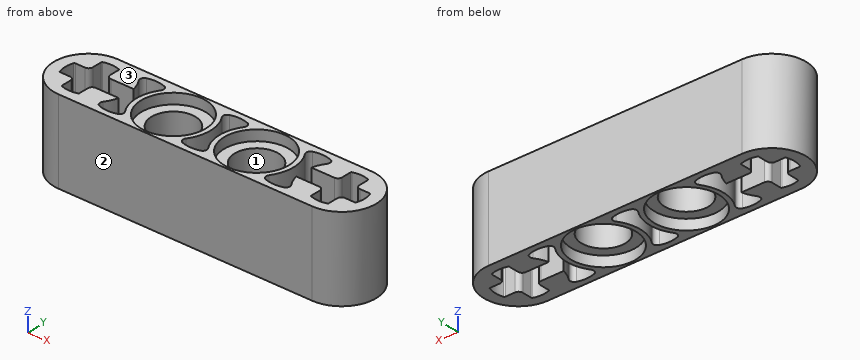
from build123d import *

# Parameters (mm, degrees)
SKETCH1_R           = 2.1
BOSS_EXTRUDE1_DEPTH = 4
SKETCH2_R           = 3.1
CUT_EXTRUDE1_DEPTH  = 1


with BuildPart() as part:
    # Sketch1 → Boss-Extrude1 (new, symmetric)
    with BuildSketch(Plane.XY):
        with BuildLine():
            Line((12.2, 3.3), (-12.2, 3.3))
            ThreePointArc((-12.2, 3.3), (-15.5, 0), (-12.2, -3.3))
            Line((-12.2, -3.3), (12.2, -3.3))
            ThreePointArc((12.2, -3.3), (15.5, 0), (12.2, 3.3))
        make_face()
        with BuildLine():
            Line((-14.177705214, 0.84), (-13.24, 0.84))
            ThreePointArc((-13.24, 0.84), (-12.957157288, 0.957157288), (-12.84, 1.24))
            Line((-12.84, 1.24), (-12.84, 2.177705214))
            ThreePointArc((-12.84, 2.177705214), (-12.821293884, 2.235940121), (-12.772173913, 2.27238805))
            ThreePointArc((-12.772173913, 2.27238805), (-12, 2.4), (-11.227826087, 2.27238805))
            ThreePointArc((-11.227826087, 2.27238805), (-11.178706116, 2.235940121), (-11.16, 2.177705214))
            Line((-11.16, 2.177705214), (-11.16, 1.24))
            ThreePointArc((-11.16, 1.24), (-11.042842712, 0.957157288), (-10.76, 0.84))
            Line((-10.76, 0.84), (-9.822294786, 0.84))
            Line((-9.822294786, 0.84), (-9.751800721, 0.84))
            Line((-9.751800721, 0.84), (-8.55081169, 0.84))
            ThreePointArc((-8.55081169, 0.84), (-8.757752494, 1.445797742), (-9.070126582, 2.004580194))
            ThreePointArc((-9.070126582, 2.004580194), (-9.119033599, 2.358251088), (-8.865957447, 2.610099174))
            ThreePointArc((-8.865957447, 2.610099174), (-8, 2.75), (-7.134042553, 2.610099174))
            ThreePointArc((-7.134042553, 2.610099174), (-6.880966401, 2.358251088), (-6.929873418, 2.004580194))
            ThreePointArc((-6.929873418, 2.004580194), (-7.55, 0), (-6.929873418, -2.004580194))
            ThreePointArc((-6.929873418, -2.004580194), (-6.880966401, -2.358251088), (-7.134042553, -2.610099174))
            ThreePointArc((-7.134042553, -2.610099174), (-8, -2.75), (-8.865957447, -2.610099174))
            ThreePointArc((-8.865957447, -2.610099174), (-9.119033599, -2.358251088), (-9.070126582, -2.004580194))
            ThreePointArc((-9.070126582, -2.004580194), (-8.757752494, -1.445797742), (-8.55081169, -0.84))
            Line((-8.55081169, -0.84), (-9.751800721, -0.84))
            Line((-9.751800721, -0.84), (-9.822294786, -0.84))
            Line((-9.822294786, -0.84), (-10.76, -0.84))
            ThreePointArc((-10.76, -0.84), (-11.042842712, -0.957157288), (-11.16, -1.24))
            Line((-11.16, -1.24), (-11.16, -2.177705214))
            ThreePointArc((-11.16, -2.177705214), (-11.178706116, -2.235940121), (-11.227826087, -2.27238805))
            ThreePointArc((-11.227826087, -2.27238805), (-12, -2.4), (-12.772173913, -2.27238805))
            ThreePointArc((-12.772173913, -2.27238805), (-12.821293884, -2.235940121), (-12.84, -2.177705214))
            Line((-12.84, -2.177705214), (-12.84, -1.24))
            ThreePointArc((-12.84, -1.24), (-12.957157288, -0.957157288), (-13.24, -0.84))
            Line((-13.24, -0.84), (-14.177705214, -0.84))
            ThreePointArc((-14.177705214, -0.84), (-14.235940121, -0.821293884), (-14.27238805, -0.772173913))
            ThreePointArc((-14.27238805, -0.772173913), (-14.4, 0), (-14.27238805, 0.772173913))
            ThreePointArc((-14.27238805, 0.772173913), (-14.235940121, 0.821293884), (-14.177705214, 0.84))
        make_face(mode=Mode.SUBTRACT)
        with BuildLine():
            ThreePointArc((0.865957447, -2.610099174), (0, -2.75), (-0.865957447, -2.610099174))
            ThreePointArc((-0.865957447, -2.610099174), (-1.119033599, -2.358251088), (-1.070126582, -2.004580194))
            ThreePointArc((-1.070126582, -2.004580194), (-0.45, 0), (-1.070126582, 2.004580194))
            ThreePointArc((-1.070126582, 2.004580194), (-1.119033599, 2.358251088), (-0.865957447, 2.610099174))
            ThreePointArc((-0.865957447, 2.610099174), (0, 2.75), (0.865957447, 2.610099174))
            ThreePointArc((0.865957447, 2.610099174), (1.119033599, 2.358251088), (1.070126582, 2.004580194))
            ThreePointArc((1.070126582, 2.004580194), (0.45, 0), (1.070126582, -2.004580194))
            ThreePointArc((1.070126582, -2.004580194), (1.119033599, -2.358251088), (0.865957447, -2.610099174))
        make_face(mode=Mode.SUBTRACT)
        with BuildLine():
            Line((12.84, 2.177705214), (12.84, 1.24))
            ThreePointArc((12.84, 1.24), (12.957157288, 0.957157288), (13.24, 0.84))
            Line((13.24, 0.84), (14.177705214, 0.84))
            ThreePointArc((14.177705214, 0.84), (14.235940121, 0.821293884), (14.27238805, 0.772173913))
            ThreePointArc((14.27238805, 0.772173913), (14.4, 0), (14.27238805, -0.772173913))
            ThreePointArc((14.27238805, -0.772173913), (14.235940121, -0.821293884), (14.177705214, -0.84))
            Line((14.177705214, -0.84), (13.24, -0.84))
            ThreePointArc((13.24, -0.84), (12.957157288, -0.957157288), (12.84, -1.24))
            Line((12.84, -1.24), (12.84, -2.177705214))
            ThreePointArc((12.84, -2.177705214), (12.821293884, -2.235940121), (12.772173913, -2.27238805))
            ThreePointArc((12.772173913, -2.27238805), (12, -2.4), (11.227826087, -2.27238805))
            ThreePointArc((11.227826087, -2.27238805), (11.178706116, -2.235940121), (11.16, -2.177705214))
            Line((11.16, -2.177705214), (11.16, -1.24))
            ThreePointArc((11.16, -1.24), (11.042842712, -0.957157288), (10.76, -0.84))
            Line((10.76, -0.84), (9.822294786, -0.84))
            Line((9.822294786, -0.84), (9.751800721, -0.84))
            Line((9.751800721, -0.84), (8.55081169, -0.84))
            ThreePointArc((8.55081169, -0.84), (8.757752494, -1.445797742), (9.070126582, -2.004580194))
            ThreePointArc((9.070126582, -2.004580194), (9.119033599, -2.358251088), (8.865957447, -2.610099174))
            ThreePointArc((8.865957447, -2.610099174), (8, -2.75), (7.134042553, -2.610099174))
            ThreePointArc((7.134042553, -2.610099174), (6.880966401, -2.358251088), (6.929873418, -2.004580194))
            ThreePointArc((6.929873418, -2.004580194), (7.55, 0), (6.929873418, 2.004580194))
            ThreePointArc((6.929873418, 2.004580194), (6.880966401, 2.358251088), (7.134042553, 2.610099174))
            ThreePointArc((7.134042553, 2.610099174), (8, 2.75), (8.865957447, 2.610099174))
            ThreePointArc((8.865957447, 2.610099174), (9.119033599, 2.358251088), (9.070126582, 2.004580194))
            ThreePointArc((9.070126582, 2.004580194), (8.757752494, 1.445797742), (8.55081169, 0.84))
            Line((8.55081169, 0.84), (9.751800721, 0.84))
            Line((9.751800721, 0.84), (9.822294786, 0.84))
            Line((9.822294786, 0.84), (10.76, 0.84))
            ThreePointArc((10.76, 0.84), (11.042842712, 0.957157288), (11.16, 1.24))
            Line((11.16, 1.24), (11.16, 2.177705214))
            ThreePointArc((11.16, 2.177705214), (11.178706116, 2.235940121), (11.227826087, 2.27238805))
            ThreePointArc((11.227826087, 2.27238805), (12, 2.4), (12.772173913, 2.27238805))
            ThreePointArc((12.772173913, 2.27238805), (12.821293884, 2.235940121), (12.84, 2.177705214))
        make_face(mode=Mode.SUBTRACT)
        with Locations((-4, 0)):
            Circle(SKETCH1_R, mode=Mode.SUBTRACT)
        with Locations((4, 0)):
            Circle(SKETCH1_R, mode=Mode.SUBTRACT)
    extrude(amount=BOSS_EXTRUDE1_DEPTH, both=True)

    # Sketch2 → Cut-Extrude1 (cut)
    with BuildSketch(Plane.XY.offset(4)):
        with Locations((-4, 0)):
            Circle(SKETCH2_R)
        with Locations((4, 0)):
            Circle(SKETCH2_R)
    cut_extrude1 = extrude(amount=-CUT_EXTRUDE1_DEPTH, mode=Mode.SUBTRACT)

    # Mirror1: Cut-Extrude1 across plane
    add(cut_extrude1.mirror(Plane.XY), mode=Mode.SUBTRACT)


solid = part.part
Design review of the part built by this model. Coordinates are the model's own, in mm. Face numbers are marked on the shaded views. Round coordinates to 2 decimals unless told otherwise and drop trailing zeros. Write each loop counter-clockwise with the first axis right and the second up, starting at its lowest first coordinate (ties: lowest second). Pieces come first, ordered by that corner, then holes. Notation, with made-up numbers: (-26, 13) - (-22, 13) arc R26 ccw to (-22, 32) - close; hole circle Ø5 at (-25, 21). An arc over 180 degrees is marked (long way). Use a Markdown table: item, result. Add a question column.
1. We need section B-B (z = 1.75). Count the separate pieces of the cut face and the enclosed holes in it, then the cut area to 3 significant figures.
2. Mouldability with a two-part tool opening along Y and no side actions: class the marked faces 1, 2 and 3 as +Y half, -Y half, draft (parallel to the pull), parting line (faces both ways), or undercut.
3. Clearance check with flat-ended pins moving along their axes: pin 1 (2 mm diameter, centred on x = 12.5, y = -0.5, fed in from +Z); pin 2 (0.5 mm diameter, centred on y = -1.5, z = 2, fed in from +X); pin 3 (1 mm diameter, centred on x = 13.5, z = 0.5, fed in from +Y); pin 4 (0.5 mm diameter, centred on x = 13.5, z = 0, fed in from -Y). State where each tip first meets the part, or that it passes through.
4. We need section A-A (x = 4). State the section outline as (y, z) points, then the cut area to 3 significant figures.
5. We need section C-C (x = -9.5). State the section outline as (y, z) points.
6. Wall thickness on probe 1 along Y at (x, z) = (-4, -3.4); probe 2 along Y at (x, z) = (-7, -1); probe 3 along X at (y, z) = (0.75, 1.75): over which ranges is each line inside the solid? List them lowest first.
Output:
| question | item | result |
|---|---|---|
| 1 | separate pieces | 1 |
| 1 | enclosed holes | 5 |
| 1 | area | 113 mm2 |
| 2 | face 1 | undercut |
| 2 | face 2 | -Y half |
| 2 | face 3 | draft |
| 3 | pin 1 | stops at z = 4 |
| 3 | pin 2 | stops at x = 15.25 |
| 3 | pin 3 | stops at y = 3.2 |
| 3 | pin 4 | stops at y = -3.13 |
| 4 | outline | (-3.3, -4) - (-3.1, -4) - (-3.1, -3) - (-2.1, -3) - (-2.1, 3) - (-3.1, 3) - (-3.1, 4) - (-3.3, 4) - close; (2.1, -3) - (3.1, -3) - (3.1, -4) - (3.3, -4) - (3.3, 4) - (3.1, 4) - (3.1, 3) - (2.1, 3) - close |
| 4 | area | 15.2 mm2 |
| 5 | outline | (-3.3, -4) - (-0.84, -4) - (-0.84, 4) - (-3.3, 4) - close; (0.84, -4) - (3.3, -4) - (3.3, 4) - (0.84, 4) - close |
| 6 | probe 1 | y = -3.3 to -3.1, 3.1 to 3.3 |
| 6 | probe 2 | y = -3.3 to -2.53, -1.9 to 1.9, 2.53 to 3.3 |
| 6 | probe 3 | x = -15.41 to -14.28, -7.47 to -5.96, -2.04 to -0.53, 0.53 to 2.04, 5.96 to 7.47, 14.28 to 15.41 |
